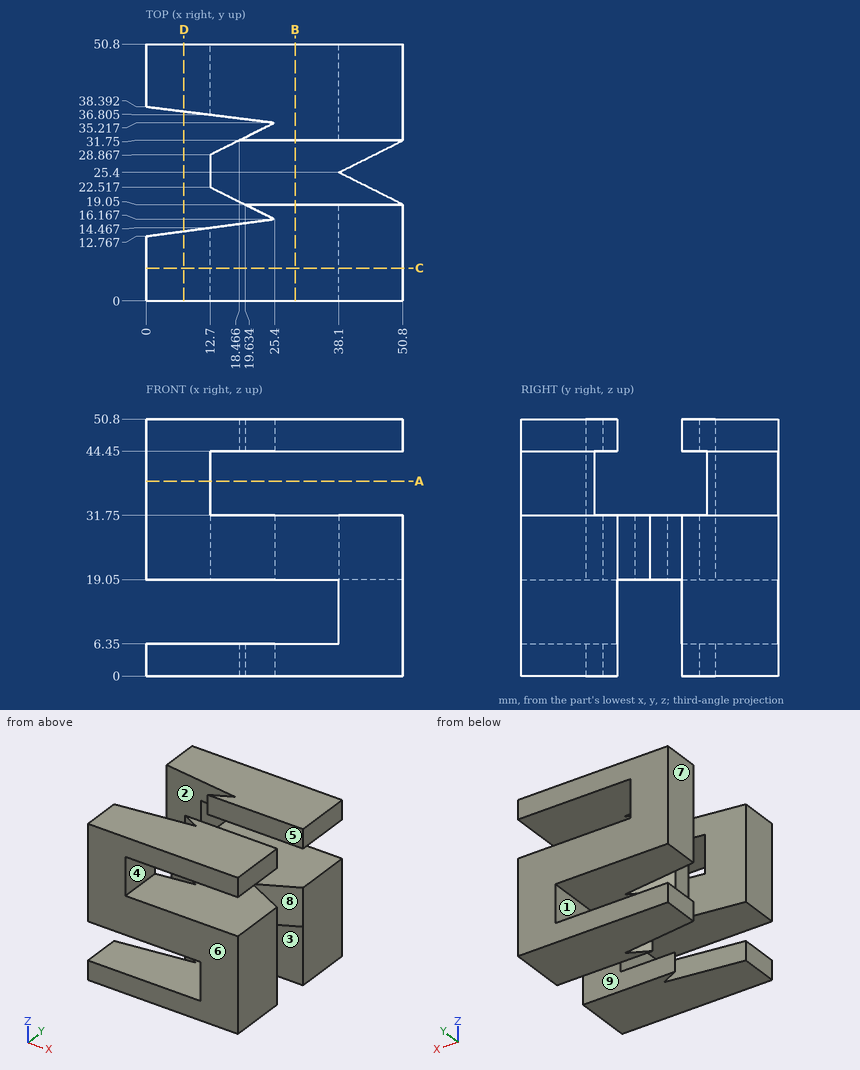
Geometry check sheet. Reference: drawing and pictorial views, mm from the part's lowest x, y, z. A direction names the side the tool comes from. Give positions to 0.01 mm unless a question says otherwise; leave off trailing zeros. Order: outer loops, then holes, each group sorted by start corner. A loop starts at its lowest first (then second) coordinate and runs counter-clockwise, first axis right, second up. Notation, with made-up numbers: M -27.75,88.25 L -0.75,88.25 A12 cw -0.75,94.25 Z; hole C -1.5,50 d1. An arc over 180 degrees is marked long. Answer in a Markdown table with one row per item. Add a question column.
Item 1: Section check B-B, the plane x = 29.5. Enter the section's corners in (y, z), and give its area (3 significant figures).
Item 2: Tool access check on the marked faces 1, 2, 3, 4 and 5. Record the directions out of +Z, -Z, +X, -X, +Y, -Y that give a thin tool (end or side, any length) a straight path to the whole face; none if there is none.
Item 3: Section check D-D, the plane x = 7.5. State how many separate pieces and enclosed holes the cut face has, and give its area (3 significant figures).
Item 4: Scan lines: probe 1 along Z at (x, y) = (32, 43.5); probe 2 along Y at (x, z) = (26, 5.5); probe 3 along Z at (x, y) = (7, 43.5). Record each from-to range of solid material in increasing order. Write a range as from..to.
Item 5: Mould release check, pull along Y, two halves, no side actions. Record for the marked faces 6, 7, 8 and 9: released by +Y, released by -Y, zero draft, split by the parting line, or undercut.
Item 6: Gauge pin test, flat ends, axial feed: pin 1 (4 mm diameter, centred on y = 43.5, z = 37, fed in from +X); pin 2 (3 mm diameter, centred on y = 25.5, z = 22, fed in from -X); pin 3 (8 mm diameter, centred on x = 30.5, y = 25, fed in from -Z); pin 4 (3 mm diameter, centred on y = 22.5, z = 13.5, fed in from +X). Record the tip position at first contact, or that the pin passes through.
Item 7: Section check C-C, the plane y = 6.5. Enter the section's corners in (x, z).
Item 8: Section check A-A, the plane z = 38.5. Enter the section's corners in (x, y) (1 decimal).
Filled sheet:
| question | item | result |
|---|---|---|
| 1 | outline | M 0,0 L 19.05,0 L 19.05,6.35 L 0,6.35 Z; M 0,19.05 L 50.8,19.05 L 50.8,31.75 L 0,31.75 Z; M 0,44.45 L 19.05,44.45 L 19.05,50.8 L 0,50.8 Z; M 31.75,0 L 50.8,0 L 50.8,6.35 L 31.75,6.35 Z; M 31.75,44.45 L 50.8,44.45 L 50.8,50.8 L 31.75,50.8 Z |
| 1 | area | 1,130 mm^2 |
| 2 | face 1 | -X, +Y, -Y |
| 2 | face 2 | +Z, -Z, -X |
| 2 | face 3 | -Z, +X, -X |
| 2 | face 4 | +X, +Y, -Y |
| 2 | face 5 | +Z, +X, -X |
| 3 | separate pieces | 4 |
| 3 | enclosed holes | 0 |
| 3 | area | 1,030 mm^2 |
| 4 | probe 1 | z = 0..6.35, 19.05..31.75, 44.45..50.8 |
| 4 | probe 2 | y = 0..19.05, 31.75..50.8 |
| 4 | probe 3 | z = 0..6.35, 19.05..50.8 |
| 5 | face 6 | released by -Y |
| 5 | face 7 | zero draft |
| 5 | face 8 | undercut |
| 5 | face 9 | undercut |
| 6 | pin 1 | stops at x = 12.7 |
| 6 | pin 2 | stops at x = 12.7 |
| 6 | pin 3 | stops at z = 19.05 |
| 6 | pin 4 | passes through |
| 7 | outline | M 0,0 L 50.8,0 L 50.8,31.75 L 12.7,31.75 L 12.7,44.45 L 50.8,44.45 L 50.8,50.8 L 0,50.8 L 0,19.05 L 38.1,19.05 L 38.1,6.35 L 0,6.35 Z |
| 8 | outline | M 0,0 L 12.7,0 L 12.7,14.5 L 0,12.8 Z; M 0,38.4 L 12.7,36.8 L 12.7,50.8 L 0,50.8 Z |
